Design review of the part built by this model. Coordinates are the model's own, in mm. A direction names the side the tool comes from. Give positions to 0.01 mm unless a question says otherwise; leave off trailing zeros. Order: outer loops, then holes, each group sorted by start corner. A loop starts at its lowest first (then second) coordinate and runs counter-clockwise, first axis right, second up. Notation, with made-up numbers: (-15.75, 89.5) -> (43.25, 89.5) arc R14 cw to (43.25, 101.5) -> close; hole circle Ø8 at (13, -14.75). An arc over 180 degrees is marked (long way). Return JSON: item names as keys, results as strings.
```python
from build123d import *

# Parameters (mm, degrees)
F0_R     = 19
F1_DEPTH = 24
F2_R     = 11
F3_DEPTH = 7
F4_R     = 11
F5_DEPTH = 7
F6_R     = 29.5
F6_R_2   = 19
F7_DEPTH = 36
F8_SIZE  = 10


with BuildPart() as f1:
    # F0 (on Top) → F1 (new body)
    with BuildSketch(Plane.XY):
        Circle(F0_R)
        with BuildLine():
            ThreePointArc((-9.5262794416, 5.5), (-5.5, 9.5262794416), (0, 11))
            ThreePointArc((0, 11), (5.5, 9.5262794416), (9.5262794416, 5.5))
            ThreePointArc((9.5262794416, 5.5), (10.6251840892, 2.8470094961), (11, 0))
            ThreePointArc((11, 0), (10.6251840892, -2.8470094961), (9.5262794416, -5.5))
            ThreePointArc((9.5262794416, -5.5), (5.5, -9.5262794416), (0, -11))
            ThreePointArc((0, -11), (-5.5, -9.5262794416), (-9.5262794416, -5.5))
            ThreePointArc((-9.5262794416, -5.5), (-11, 0), (-9.5262794416, 5.5))
        make_face(mode=Mode.SUBTRACT)
        with BuildLine():
            ThreePointArc((11, 0), (10.6251840892, 2.8470094961), (9.5262794416, 5.5))
            Line((9.5262794416, 5.5), (8.6602540378, 5))
            ThreePointArc((8.6602540378, 5), (10, 0), (8.6602540378, -5))
            Line((8.6602540378, -5), (9.5262794416, -5.5))
            ThreePointArc((9.5262794416, -5.5), (10.6251840892, -2.8470094961), (11, 0))
        make_face()
        with BuildLine():
            ThreePointArc((-8.6602540378, 5), (-5, 8.6602540378), (0, 10))
            Line((0, 10), (0, 11))
            ThreePointArc((0, 11), (-5.5, 9.5262794416), (-9.5262794416, 5.5))
            Line((-9.5262794416, 5.5), (-8.6602540378, 5))
        make_face()
        with BuildLine():
            Line((-8.6602540378, -5), (-9.5262794416, -5.5))
            ThreePointArc((-9.5262794416, -5.5), (-5.5, -9.5262794416), (0, -11))
            Line((0, -11), (0, -10))
            ThreePointArc((0, -10), (-5, -8.6602540378), (-8.6602540378, -5))
        make_face()
    extrude(amount=F1_DEPTH)

    # F2 (on Top) → F3 (cut)
    with BuildSketch(Plane.XY):
        Circle(F2_R)
    extrude(amount=F3_DEPTH, mode=Mode.SUBTRACT)

    # F4 (on face) → F5 (cut)
    with BuildSketch(Plane.XY.offset(24)):
        Circle(F4_R)
    extrude(amount=-F5_DEPTH, mode=Mode.SUBTRACT)

    # F6 (on Top) → F7 (join)
    with BuildSketch(Plane.XY):
        Circle(F6_R)
        Circle(F6_R_2, mode=Mode.SUBTRACT)
    extrude(amount=F7_DEPTH)

    # F8
    f8_edges = [f1.edges().sort_by_distance(p)[0] for p in [
        (-19, 0, 36),
    ]]
    chamfer(f8_edges, length=F8_SIZE)


solid = f1.part
```
Item 1: Add section C-C (z = 21). Give the boundary of the cut face in (x, y).
Result set:
{"outline": "circle Ø59 at (0, 0); hole circle Ø22 at (0, 0)"}
Item 2: For pin 1 (1.5 mm diameter, centred on y = -16, z = 12, fed in from +X); pin 2 (5 mm diameter, centred on y = 9, z = 9.5, fed in from -X) (3 decimals); pin 3 (0.8 mm diameter, centred on y = 10.5, z = 13, fed in from +X), all flat-tipped, find the tip position at first contact; note any pin that passes through.
Result set:
{"pin 1": "stops at x = 25.25", "pin 2": "stops at x = -28.775", "pin 3": "stops at x = 27.72"}
Item 3: Mouldability with a two-part tool opening along X and no side actions: class faces 1 (the face through (21.7, -19.5, 36)), 2 (the face through (10, 0, 12)), 3 (the face through (8.767, -16.856, 24.986)), 4 (the face through (28.14, 8.86, 17.75)) as released by +X, released by -X, zero draft, split by the parting line, or undercut.
Result set:
{"face 1": "zero draft", "face 2": "undercut", "face 3": "undercut", "face 4": "split by the parting line"}
Item 4: Add section D-D (z = 25). Give the boundary of the cut face in (x, y).
Result set:
{"outline": "circle Ø59 at (0, 0); hole circle Ø38 at (0, 0)"}
Item 5: Add section B-B (y = 0). Give the boundary of the cut face in (x, z), plus the area to 3 significant figures.
Result set:
{"outline": "(-29.5, 0) -> (-11, 0) -> (-11, 24) -> (-19, 24) -> (-19, 26) -> (-29, 36) -> (-29.5, 36) -> close; (10, 7) -> (11, 7) -> (11, 0) -> (29.5, 0) -> (29.5, 36) -> (29, 36) -> (19, 26) -> (19, 24) -> (11, 24) -> (11, 17) -> (10, 17) -> close", "area": "1,050 mm^2"}
Item 6: Add section A-A (z = 9). Give the boundary of the cut face in (x, y), plus the area to 3 significant figures.
Result set:
{"outline": "circle Ø59 at (0, 0); hole (-9.53, -5.5) -> (-8.66, -5) arc R10 ccw to (0, -10) -> (0, -11) arc R11 ccw to (9.53, -5.5) -> (8.66, -5) arc R10 ccw to (8.66, 5) -> (9.53, 5.5) arc R11 ccw to (0, 11) -> (0, 10) arc R10 ccw to (-8.66, 5) -> (-9.53, 5.5) arc R11 ccw to start", "area": "2,390 mm^2"}
Item 7: Wall thickness on L1, parallel to Y at x = 0, z = 25.4; L2, parallel to X at y = 9, z = 27; L3, parallel to X at y = 10, z = 32.5: over which ranges is each line inside the solid? List them lowest first. Write a range as [from, to].
Result set:
{"L1": "y = [-29.5, -19], [19, 29.5]", "L2": "x = [-28.09, -17.86], [17.86, 28.09]", "L3": "x = [-27.75, -23.46], [23.46, 27.75]"}
Item 8: Machinability: for faces 5 (the face through (10.3, 0.1, 7)), 6 (the face through (-5, -9, 17)), 7 (the face through (-5.1, 8.6, 11.9)), 8 (the face through (0, -13, 0)), which of the approach directions +Z, -Z, +X, -X, +Y, -Y give a long, thin tool a straight path to every point of the face, cutting with its end or side? Answer none if there is none.
Result set:
{"face 5": "-Z", "face 6": "+Z", "face 7": "+Z, -Z", "face 8": "-Z, +X, -X, +Y, -Y"}
